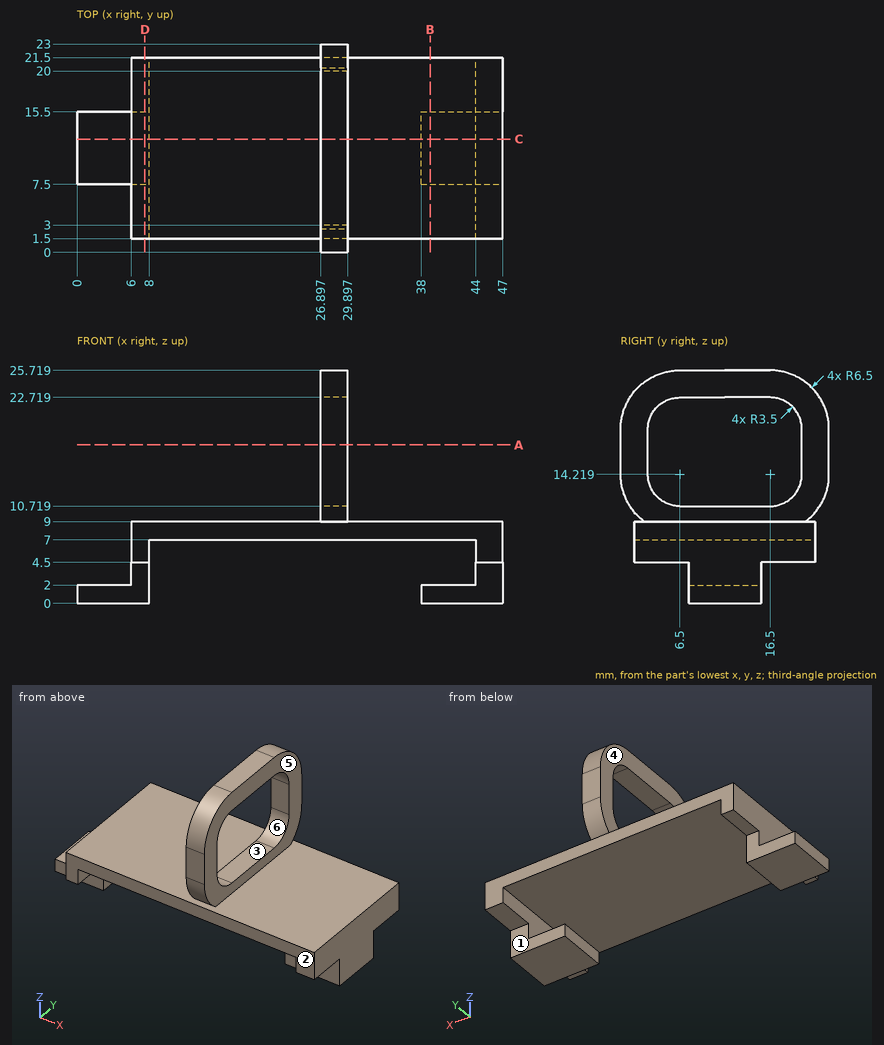
Design review of the part shown in the three views and the two pictorial views. Dimensions are in mm from the part's minimum x, y and z. A direction names the side the tool comes from. Round coordinates to 2 decimals unless told otherwise and drop trailing zeros. Write each loop counter-clockwise with the first axis right and the second up, starting at its lowest first coordinate (ties: lowest second). Pieces come first, ordered by that corner, then holes. Notation, with made-up numbers: (61.5, 80.5) - (117.5, 80.5) arc R28 ccw to (117.5, 107.5) - close; hole circle Ø2 at (54.5, 52). An arc over 180 degrees is marked (long way). Answer as CSV lines item,"result". Start each with the question number.
(1) Add section A-A, the plane z = 17.5. State the section outline as (x, y) points, plus the area to 3 significant figures.
(2) Add section B-B, the plane x = 39. State the section outline as (y, z) points, plus the area to 3 significant figures.
(3) Mouldability with a two-part tool opening along Y and no side actions: class the marked faces 1, 2 and 3 as +Y half, -Y half, draft (parallel to the pull), parting line (faces both ways), or undercut.
(4) For pin 1 (1.5 mm diameter, centred on y = 4.5, z = 22, fed in from +X); pin 2 (10 mm diameter, centred on x = 32, y = 15, fed in from -Z); pin 3 (4 mm diameter, centred on y = 12, z = 4.5, fed in from -X), all flat-tipped, find the tip position at first contact; note any pin that passes through.
(5) Add section C-C, the plane y = 12.5. State the section outline as (x, z) points.
(6) Add section D-D, the plane x = 7.5. State the section outline as (y, z) points.
(7) Machinability: for the marked faces 4, 5 and 6, which of the approach directions +Z, -Z, +X, -X, +Y, -Y give a long, thin tool a straight path to every point of the face, cutting with its end or side? Answer none if there is none.
(8) For line 1 (Z direction, x = 41, y = 12.25); line 2 (Z direction, x = 27, y = 6.75); line 3 (X direction, y = 8, z = 7.25), list the stretches that pass through material, from the lowest coordinate up.
From the geometry:
1,outline,"(26.9, 0) - (29.9, 0) - (29.9, 3) - (26.9, 3) - close; (26.9, 20) - (29.9, 20) - (29.9, 23) - (26.9, 23) - close"
1,area,"18.0 mm²"
2,outline,"(1.5, 7) - (21.5, 7) - (21.5, 9) - (1.5, 9) - close; (7.5, 0) - (15.5, 0) - (15.5, 2) - (7.5, 2) - close"
2,area,"56.0 mm²"
3,face 1,"+Y half"
3,face 2,"-Y half"
3,face 3,"undercut"
4,pin 1,"stops at x = 29.9"
4,pin 2,"stops at z = 7"
4,pin 3,"stops at x = 6"
5,outline,"(0, 0) - (8, 0) - (8, 7) - (44, 7) - (44, 2) - (38, 2) - (38, 0) - (47, 0) - (47, 9) - (29.9, 9) - (29.9, 10.72) - (26.9, 10.72) - (26.9, 9) - (6, 9) - (6, 2) - (0, 2) - close; (26.9, 22.72) - (29.9, 22.72) - (29.9, 25.72) - (26.9, 25.72) - close"
6,outline,"(1.5, 4.5) - (7.5, 4.5) - (7.5, 0) - (15.5, 0) - (15.5, 4.5) - (21.5, 4.5) - (21.5, 9) - (1.5, 9) - close"
7,face 4,"+Z, -X, +Y, -Y"
7,face 5,"+Z, +X, +Y, -Y"
7,face 6,"+X, -X"
8,line 1,"z = 0 to 2, 7 to 9"
8,line 2,"z = 7 to 10.72, 22.72 to 25.72"
8,line 3,"x = 6 to 47"
